Verification items for the finished model (mm, model axes). A direction names the side the tool comes from. Round coordinates to 2 decimals unless told otherwise and drop trailing zeros. Order: outer loops, then holes, each group sorted by start corner. A loop starts at its lowest first (then second) coordinate and runs counter-clockwise, first axis right, second up.
```python
from build123d import *

# Parameters (mm, degrees)
F0_W     = 105.4313331842
F0_H     = 68.6848964542
F1_DEPTH = 127
F2_DEPTH = 25.4
F3_W     = 105.4313331842
F3_H     = 38.4183302522
F4_DEPTH = 94.488
F5_W     = 18.094740808
F5_H     = 17.1922501177
F5_W_2   = 18.4211255983
F5_H_2   = 13.3941207528
F6_DEPTH = 112.014


with BuildPart() as f1:
    # F0 (on Front) → F1 (new body)
    with BuildSketch(Plane.XZ):
        with Locations((-19.3043276668, -17.4522669986)):
            Rectangle(F0_W, F0_H)
    extrude(amount=F1_DEPTH)

    # F2 (cut): a face of the model
    f2_faces = [f1.faces().sort_by_distance(p)[0] for p in [
        (-19.3043276668, -63.5, 16.8901812285),
    ]]
    extrude(f2_faces, amount=-F2_DEPTH, mode=Mode.SUBTRACT)

    # F3 (on face) → F4 (join)
    with BuildSketch(Plane.XY.offset(-8.5098187715)):
        with Locations((-19.3043276668, -19.2091651261)):
            Rectangle(F3_W, F3_H)
    extrude(amount=F4_DEPTH)

    # F5 (on face) → F6 (join)
    with BuildSketch(Plane(origin=(0, 0, -51.7947152257), x_dir=(1, 0, 0), z_dir=(0, 0, -1))):
        with Locations((-62.9726238549, 8.5961250588)):
            Rectangle(F5_W, F5_H)
        with Locations((24.2007761262, 8.5961250588)):
            Rectangle(F5_W_2, F5_H)
        with Locations((24.2007761262, 120.3029396236)):
            Rectangle(F5_W_2, F5_H_2)
        with Locations((-62.9726238549, 120.3029396236)):
            Rectangle(F5_W, F5_H_2)
    extrude(amount=F6_DEPTH)


solid = f1.part
```
1) Scan lines: probe 1 along Y at (x, z) = (26.5, -87.5); probe 2 along X at (y, z) = (-9, -95); probe 3 along Z at (x, y) = (-2.5, -92.5). Record each from-to range of solid material in increasing order.
2) Draft check along X on faces 4 (the flat face through (14.99, -8, -107)), 5 (the flat face through (-20, -127, -51)), 6 (the flat face through (33.411, -50, -41)), 7 (the flat face through (-53.925, -8, -107)). Enter one of: released by +X, released by -X, zero draft, split by the parting line, or undercut.
3) Sectioned sample at D-D on y = -78.5. Record the cut outline in (x, z).
4) Go/stop test with flat-tipped pins: pin 1 Ø2 at (x, z) = (-25.5, 52) entering from -Y; pin 2 Ø4 at (x, y) = (13.5, -47) entering from +Z; pin 3 Ø6 at (x, y) = (-48, -87) entering from -Z. Record where each tip stops, or that it passes through.
5) Sectioned sample at B-B on x = -8.5. Record the cut outline in (y, z).
6) Sectioned sample at A-A on z = -129.5. Record the cut outline in (x, y).
7) Sectioned sample at C-C on x = -59.5. Record the cut outline in (y, z), then the cut area to 3 significant figures.
8) Tool access check on faces 1 (the flat face through (14.99, -120, -107)), 2 (the flat face through (-20, -38.418, 38)), 3 (the flat face through (-63, -113.606, -107)). Record the directions out of +Z, -Z, +X, -X, +Y, -Y that give a thin tool (end or side, any length) a straight path to the whole face; none if there is none.
Returned:
1. probe 1: y = -127 to -113.61, -17.19 to 0
1. probe 2: x = -72.02 to -53.93, 14.99 to 33.41
1. probe 3: z = -51.79 to -8.51
2. face 4: undercut
2. face 5: zero draft
2. face 6: released by +X
2. face 7: undercut
3. outline: (-72.02, -51.79) - (33.41, -51.79) - (33.41, -8.51) - (-72.02, -8.51) - close
4. pin 1: stops at y = -38.42
4. pin 2: stops at z = -8.51
4. pin 3: stops at z = -51.79
5. outline: (-127, -51.79) - (0, -51.79) - (0, 85.98) - (-38.42, 85.98) - (-38.42, -8.51) - (-127, -8.51) - close
6. outline: (-72.02, -127) - (-53.93, -127) - (-53.93, -113.61) - (-72.02, -113.61) - close; (-72.02, -17.19) - (-53.93, -17.19) - (-53.93, 0) - (-72.02, 0) - close; (14.99, -127) - (33.41, -127) - (33.41, -113.61) - (14.99, -113.61) - close; (14.99, -17.19) - (33.41, -17.19) - (33.41, 0) - (14.99, 0) - close
7. outline: (-127, -163.81) - (-113.61, -163.81) - (-113.61, -51.79) - (-17.19, -51.79) - (-17.19, -163.81) - (0, -163.81) - (0, 85.98) - (-38.42, 85.98) - (-38.42, -8.51) - (-127, -8.51) - close
7. area: 12,600 mm2
8. face 1: -Z, +Y, -Y
8. face 2: +Z, +X, -X, -Y
8. face 3: -Z, +X, -X
